Source: CAD feature listing. Evaluate the final solid. Frame: model axes, mm. Face numbers are marked on the shaded views. A direction names the side the tool comes from. Give positions to 0.01 mm unless a question says otherwise; leave off trailing zeros. Loops run counter-clockwise (first coordinate to the right, second up) from the corner with the lowest first, then second, coordinate; pieces in that order, holes last. Notation, with made-up numbers: (-2.75, -35.5) - (51.25, -35.5) arc R20 ccw to (51.25, -21.5) - close; hole circle Ø11 at (-3, -2.75). An arc over 180 degrees is marked (long way). Put each result on its own line as item: value.
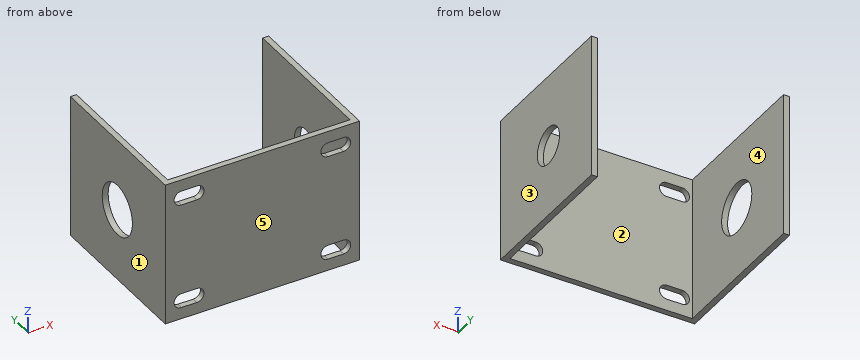
```python
from build123d import *

# Parameters (mm, degrees)
SKETCH1_W               = 1
SKETCH1_H               = 25.7
SKETCH1_H_2             = 1
SKETCH1_W_2             = 30.5
SKETCH1_H_3             = 24.613793103
BOSS_EXTRUDE1_DEPTH     = 12
CUT_EXTRUDE1_DEPTH      = 44.43604494
CUT_EXTRUDE1_DEPTH_BACK = 44.43604494
SKETCH2_R               = 3.125
CUT_EXTRUDE2_DEPTH      = 44.43604494
CUT_EXTRUDE2_DEPTH_BACK = 24
SKETCH3_R               = 4.25
CUT_EXTRUDE3_DEPTH      = 24


with BuildPart() as part:
    # Sketch1 → Boss-Extrude1 (new, symmetric)
    with BuildSketch(Plane.XY):
        with Locations((-15.75, 13.35)):
            Rectangle(SKETCH1_W, SKETCH1_H)
        with Locations((-15.75, 0)):
            Rectangle(SKETCH1_W, SKETCH1_H_2)
        Rectangle(SKETCH1_W_2, SKETCH1_H_2)
        with Locations((15.75, 0)):
            Rectangle(SKETCH1_W, SKETCH1_H_2)
        with Locations((15.75, 12.806896552)):
            Rectangle(SKETCH1_W, SKETCH1_H_3)
    extrude(amount=BOSS_EXTRUDE1_DEPTH, both=True)

    # Sketch2 → Cut-Extrude1 (cut, two sides: drawn at the far end of the back side and taken through both)
    with BuildSketch(Plane(origin=(16.25, 0, 0), x_dir=(0, 0, -1), z_dir=(1, 0, 0)).offset(-CUT_EXTRUDE1_DEPTH_BACK)):
        with Locations((0, 13)):
            Circle(SKETCH2_R)
    extrude(amount=CUT_EXTRUDE1_DEPTH + CUT_EXTRUDE1_DEPTH_BACK, mode=Mode.SUBTRACT)

    # Sketch3 → Cut-Extrude2 (cut, two sides: drawn at the far end of the back side and taken through both)
    with BuildSketch(Plane.ZY.offset(16.25).offset(-CUT_EXTRUDE2_DEPTH_BACK)):
        with Locations(Location((0, 13, 0), (0, 0, 90))):
            Circle(SKETCH3_R)
    extrude(amount=CUT_EXTRUDE2_DEPTH + CUT_EXTRUDE2_DEPTH_BACK, mode=Mode.SUBTRACT)

    # Sketch4 → Cut-Extrude3 (cut)
    with BuildSketch(Plane.XZ.offset(0.5)):
        with BuildLine():
            ThreePointArc((-13.57, -7.67), (-14.77, -8.87), (-13.57, -10.07))
            Line((-13.57, -10.07), (-13.57, -7.67))
        make_face()
        with BuildLine():
            Line((-13.57, -7.67), (-13.57, -10.07))
            ThreePointArc((-13.57, -10.07), (-12.721471863, -9.718528137), (-12.37, -8.87))
            ThreePointArc((-12.37, -8.87), (-12.721471863, -8.021471863), (-13.57, -7.67))
        make_face()
        with BuildLine():
            Line((-13.57, -10.07), (-10.97, -10.07))
            ThreePointArc((-10.97, -10.07), (-12.17, -8.87), (-10.97, -7.67))
            Line((-10.97, -7.67), (-13.57, -7.67))
            ThreePointArc((-13.57, -7.67), (-12.721471863, -8.021471863), (-12.37, -8.87))
            ThreePointArc((-12.37, -8.87), (-12.721471863, -9.718528137), (-13.57, -10.07))
        make_face()
        with BuildLine():
            ThreePointArc((-10.97, -7.67), (-12.17, -8.87), (-10.97, -10.07))
            Line((-10.97, -10.07), (-10.97, -7.67))
        make_face()
        with BuildLine():
            Line((-10.97, -7.67), (-10.97, -10.07))
            ThreePointArc((-10.97, -10.07), (-10.121471863, -9.718528137), (-9.77, -8.87))
            ThreePointArc((-9.77, -8.87), (-10.121471863, -8.021471863), (-10.97, -7.67))
        make_face()
        with BuildLine():
            ThreePointArc((10.97, -7.67), (9.77, -8.87), (10.97, -10.07))
            Line((10.97, -10.07), (10.97, -7.67))
        make_face()
        with BuildLine():
            Line((10.97, -7.67), (10.97, -10.07))
            ThreePointArc((10.97, -10.07), (11.818528137, -9.718528137), (12.17, -8.87))
            ThreePointArc((12.17, -8.87), (11.818528137, -8.021471863), (10.97, -7.67))
        make_face()
        with BuildLine():
            Line((10.97, -10.07), (13.57, -10.07))
            ThreePointArc((13.57, -10.07), (12.37, -8.87), (13.57, -7.67))
            Line((13.57, -7.67), (10.97, -7.67))
            ThreePointArc((10.97, -7.67), (11.818528137, -8.021471863), (12.17, -8.87))
            ThreePointArc((12.17, -8.87), (11.818528137, -9.718528137), (10.97, -10.07))
        make_face()
        with BuildLine():
            ThreePointArc((13.57, -7.67), (12.37, -8.87), (13.57, -10.07))
            Line((13.57, -10.07), (13.57, -7.67))
        make_face()
        with BuildLine():
            Line((13.57, -7.67), (13.57, -10.07))
            ThreePointArc((13.57, -10.07), (14.418528137, -9.718528137), (14.77, -8.87))
            ThreePointArc((14.77, -8.87), (14.418528137, -8.021471863), (13.57, -7.67))
        make_face()
        with BuildLine():
            ThreePointArc((12.17, 8.87), (11.818528137, 9.718528137), (10.97, 10.07))
            Line((10.97, 10.07), (10.97, 7.67))
            ThreePointArc((10.97, 7.67), (11.818528137, 8.021471863), (12.17, 8.87))
        make_face()
        with BuildLine():
            Line((10.97, 7.67), (10.97, 10.07))
            ThreePointArc((10.97, 10.07), (9.77, 8.87), (10.97, 7.67))
        make_face()
        with BuildLine():
            Line((13.57, 10.07), (10.97, 10.07))
            ThreePointArc((10.97, 10.07), (11.818528137, 9.718528137), (12.17, 8.87))
            ThreePointArc((12.17, 8.87), (11.818528137, 8.021471863), (10.97, 7.67))
            Line((10.97, 7.67), (13.57, 7.67))
            ThreePointArc((13.57, 7.67), (12.37, 8.87), (13.57, 10.07))
        make_face()
        with BuildLine():
            ThreePointArc((14.77, 8.87), (14.418528137, 9.718528137), (13.57, 10.07))
            Line((13.57, 10.07), (13.57, 7.67))
            ThreePointArc((13.57, 7.67), (14.418528137, 8.021471863), (14.77, 8.87))
        make_face()
        with BuildLine():
            Line((13.57, 7.67), (13.57, 10.07))
            ThreePointArc((13.57, 10.07), (12.37, 8.87), (13.57, 7.67))
        make_face()
        with BuildLine():
            ThreePointArc((-12.37, 8.87), (-12.721471863, 9.718528137), (-13.57, 10.07))
            Line((-13.57, 10.07), (-13.57, 7.67))
            ThreePointArc((-13.57, 7.67), (-12.721471863, 8.021471863), (-12.37, 8.87))
        make_face()
        with BuildLine():
            Line((-13.57, 7.67), (-13.57, 10.07))
            ThreePointArc((-13.57, 10.07), (-14.77, 8.87), (-13.57, 7.67))
        make_face()
        with BuildLine():
            Line((-10.97, 10.07), (-13.57, 10.07))
            ThreePointArc((-13.57, 10.07), (-12.721471863, 9.718528137), (-12.37, 8.87))
            ThreePointArc((-12.37, 8.87), (-12.721471863, 8.021471863), (-13.57, 7.67))
            Line((-13.57, 7.67), (-10.97, 7.67))
            ThreePointArc((-10.97, 7.67), (-12.17, 8.87), (-10.97, 10.07))
        make_face()
        with BuildLine():
            ThreePointArc((-9.77, 8.87), (-10.121471863, 9.718528137), (-10.97, 10.07))
            Line((-10.97, 10.07), (-10.97, 7.67))
            ThreePointArc((-10.97, 7.67), (-10.121471863, 8.021471863), (-9.77, 8.87))
        make_face()
        with BuildLine():
            Line((-10.97, 7.67), (-10.97, 10.07))
            ThreePointArc((-10.97, 10.07), (-12.17, 8.87), (-10.97, 7.67))
        make_face()
    extrude(amount=-CUT_EXTRUDE3_DEPTH, mode=Mode.SUBTRACT)


solid = part.part
```
1) Mould query, pull axis X, two halves, no side actions, for the marked faces 3, 4 and 5. Classes: pulls with the +X half, pulls with the -X half, needs draft (parallel to the pull), parting line crosses it, or undercut.
Check result:
face 3: pulls with the +X half
face 4: undercut
face 5: needs draft
2) Material intervals for line 1 along X through (y, z) = (15, -8.5); line 2 along Z through (x, y) = (16, 13) (3 decimals); line 3 along Z through (x, y) = (-15.5, 13), sorted ascending. Write a range as [from, to].
Check result:
line 1: [-16.25, -15.25], [15.25, 16.25]
line 2: [-12, -3.125], [3.125, 12]
line 3: [-12, -4.25], [4.25, 12]
3) Section query B-B, the plane y = 13. Output: boundary loops of the cut face in (x, z) (3 decimals).
Check result:
outline: (-16.25, -12) - (-15.25, -12) - (-15.25, -4.25) - (-16.25, -4.25) - close; (-16.25, 4.25) - (-15.25, 4.25) - (-15.25, 12) - (-16.25, 12) - close; (15.25, -12) - (16.25, -12) - (16.25, -3.125) - (15.25, -3.125) - close; (15.25, 3.125) - (16.25, 3.125) - (16.25, 12) - (15.25, 12) - close
4) Section query D-D, the plane z = -4.75. Output: boundary loops of the cut face in (x, y).
Check result:
outline: (-16.25, -0.5) - (16.25, -0.5) - (16.25, 25.11) - (15.25, 25.11) - (15.25, 0.5) - (-15.25, 0.5) - (-15.25, 26.2) - (-16.25, 26.2) - close
5) Section query C-C, the plane x = -12.5. Output: boundary loops of the cut face in (y, z), plus the area to 3 significant figures.
Check result:
outline: (-0.5, -12) - (0.5, -12) - (0.5, -10.07) - (-0.5, -10.07) - close; (-0.5, -7.67) - (0.5, -7.67) - (0.5, 7.67) - (-0.5, 7.67) - close; (-0.5, 10.07) - (0.5, 10.07) - (0.5, 12) - (-0.5, 12) - close
area: 19.2 mm²
6) Section query A-A, the plane z = 0. Output: boundary loops of the cut face in (x, y) (3 decimals), plus the area to 3 significant figures.
Check result:
outline: (-16.25, -0.5) - (16.25, -0.5) - (16.25, 9.875) - (15.25, 9.875) - (15.25, 0.5) - (-15.25, 0.5) - (-15.25, 8.75) - (-16.25, 8.75) - close; (-16.25, 17.25) - (-15.25, 17.25) - (-15.25, 26.2) - (-16.25, 26.2) - close; (15.25, 16.125) - (16.25, 16.125) - (16.25, 25.114) - (15.25, 25.114) - close
area: 68.1 mm²
7) Access query for the marked faces 1 and 2. Directions: +Z, -Z, +X, -X, +Y, -Y. A direction counts if a zero-diameter tool reaches every point of the face in a straight line with its end or side. Return the directions, or none.
Check result:
face 1: +Z, -Z, -X, +Y, -Y
face 2: +Z, -Z, +Y
8) Pin query (flat end, axial travel): P1, Ø12, axis at y = 10, z = -1, coming from the -X side; P2, Ø0.5, axis at x = 16, z = 2.5, coming from the +Y side; P3, Ø1, axis at x = -11.5, z = 0, coming from the +Y side. Return the tip coordinate at first contact, or that it passes through.
Check result:
P1: x = -16.25
P2: y = 25.11
P3: y = 0.5
